Design review of the part built by this model. Coordinates are the model's own, in mm. Give positions to 0.01 mm unless a question says otherwise; leave off trailing zeros. Loops run counter-clockwise (first coordinate to the right, second up) from the corner with the lowest first, then second, coordinate; pieces in that order, holes last. Notation, with made-up numbers: (-14.5, 13) - (30.5, 13) arc R18 cw to (30.5, 28) - close; hole circle Ø4 at (-9.75, 69.5). An arc over 180 degrees is marked (long way). Write each question's results on one line, items separated by ' | '.
from build123d import *

# Parameters (mm, degrees)
CROQUIS2_R                 = 1.5
CORTAR_EXTRUIR1_DEPTH      = 10
CROQUIS3_R                 = 1.5
SALIENTE_EXTRUIR1_DEPTH    = 3
CORTAR_EXTRUIR2_DEPTH      = 21
CORTAR_EXTRUIR2_DEPTH_BACK = 19
CROQUIS4_W                 = 22.988642253
CROQUIS4_H                 = 9.839710734
CROQUIS5_W                 = 15
CROQUIS5_H                 = 36.969240602
CORTAR_EXTRUIR3_DEPTH      = 19
CROQUIS6_W                 = 9.874263727
CROQUIS6_H                 = 12.802666517
SALIENTE_EXTRUIR2_DEPTH    = 3


with BuildPart() as part:
    # Croquis1 → Revolución1 (revolve)
    with BuildSketch(Plane.XY, mode=Mode.PRIVATE) as revoluci_n1_sk:
        Polygon((-4, 0), (-4, 7), (-5, 7), (-10.142857143, 3), (-17.142857143, 3), (-17.142857143, 0), (-14, 0), align=None)
    revolve(revoluci_n1_sk.sketch.rotate(Axis((0, 0, 0), (0, 1, 0)), 270), axis=Axis((0, 0, 0), (0, 1, 0)))

    # Croquis2 → Cortar-Extruir1 (cut)
    with BuildSketch(Plane(origin=(0, 3, 0), x_dir=(1, 0, 0), z_dir=(0, 1, 0))):
        with Locations(Location((0, 13.64, 0), (0, 0, 270))):
            Circle(CROQUIS2_R)
        with Locations(Location((13.64, 0, 0), (0, 0, 270))):
            Circle(CROQUIS2_R)
        with Locations(Location((0, -13.64, 0), (0, 0, 270))):
            Circle(CROQUIS2_R)
        with Locations(Location((-13.64, 0, 0), (0, 0, 270))):
            Circle(CROQUIS2_R)
    extrude(amount=-CORTAR_EXTRUIR1_DEPTH, mode=Mode.SUBTRACT)

    # Croquis3 → Saliente-Extruir1 (add)
    with BuildSketch(Plane(origin=(0, 3, 0), x_dir=(1, 0, 0), z_dir=(0, 1, 0))):
        with Locations((13.64, 0)):
            Circle(CROQUIS3_R)
    extrude(amount=-SALIENTE_EXTRUIR1_DEPTH)

    # Croquis4 → Cortar-Extruir2 (cut, two sides: drawn at the far end of the back side and taken through both)
    with BuildSketch(Plane.XY.offset(-CORTAR_EXTRUIR2_DEPTH_BACK)):
        with Locations((-1.351463984, 7.919855367)):
            Rectangle(CROQUIS4_W, CROQUIS4_H)
    extrude(amount=CORTAR_EXTRUIR2_DEPTH + CORTAR_EXTRUIR2_DEPTH_BACK, mode=Mode.SUBTRACT)

    # Croquis5 → Cortar-Extruir3 (cut)
    with BuildSketch(Plane(origin=(0, 3, 0), x_dir=(1, 0, 0), z_dir=(0, 1, 0))):
        with Locations((12, -0.045754011)):
            Rectangle(CROQUIS5_W, CROQUIS5_H)
    extrude(amount=-CORTAR_EXTRUIR3_DEPTH, mode=Mode.SUBTRACT)

    # Croquis6 → Saliente-Extruir2 (add)
    with BuildSketch(Plane(origin=(0, 3, 0), x_dir=(1, 0, 0), z_dir=(0, 1, 0))):
        with Locations((-0.437131864, -0.705770923)):
            Rectangle(CROQUIS6_W, CROQUIS6_H)
    extrude(amount=-SALIENTE_EXTRUIR2_DEPTH)


solid = part.part
(1) Insertion check: P1, Ø2.5, axis at x = 0, z = 13.64, coming from the -Y side. The pin has a flat end and moves straight along its axis. Give the tip position at first contact, or say it passes through.
Answers below:
P1: through
(2) Take a section at D-D on x = -14. Give the boundary of the cut face in (y, z), plus the area to 3 significant figures.
Answers below:
outline: (0, -9.89) - (3, -9.89) - (3, -1.46) - (0, -1.46) - close; (0, 1.46) - (3, 1.46) - (3, 9.89) - (0, 9.89) - close | area: 50.6 mm2
(3) Draft analysis for pull direction Z (two halves, no side actions). For faces 1 (the cylindrical face through (-17.137, 1.479, -0.441)), 2 (the flat face through (4.5, 2, 0)), 3 (the cylindrical face through (-0.575, 1.521, -12.254)), state which applies: pulls with the +Z half, pulls with the -Z half, needs draft (parallel to the pull), parting line crosses it, or undercut.
Answers below:
face 1: parting line crosses it | face 2: needs draft | face 3: undercut
(4) Wall thickness on line 1 along Z through (x, y) = (0.75, 0.6); line 2 along X through (y, z) = (0.7, 13.64); line 3 along X through (y, z) = (2.25, -14.5): over which ranges is each line inside the solid? List them lowest first. Write a range as from..to.
Answers below:
line 1: -17.13..-14.94, -12.34..12.34, 14.94..17.13 | line 2: -10.38..-1.5, 1.5..4.5 | line 3: -9.14..-1.23, 1.23..4.5
(5) Take a section at C-C on x = 0. Give the boundary of the cut face in (y, z).
Answers below:
outline: (0, -17.14) - (3, -17.14) - (3, -15.14) - (0, -15.14) - close; (0, -12.14) - (3, -12.14) - (3, 12.14) - (0, 12.14) - close; (0, 15.14) - (3, 15.14) - (3, 17.14) - (0, 17.14) - close
(6) Take a section at B-B on y = 1.95. Give the boundary of the cut face in (x, z), plus the area to 3 significant figures.
Answers below:
outline: (4.5, -16.54) - (4.5, 16.54) arc R17.14 ccw (long way) to start; hole circle Ø3 at (-13.64, 0); hole circle Ø3 at (0, -13.64); hole circle Ø3 at (0, 13.64) | area: 593 mm2
(7) Take a section at A-A on z = 0. Give the boundary of the cut face in (x, y), plus the area to 3 significant figures.
Answers below:
outline: (-17.14, 0) - (-15.14, 0) - (-15.14, 3) - (-17.14, 3) - close; (-12.14, 0) - (4.5, 0) - (4.5, 3) - (-12.14, 3) - close | area: 55.9 mm2
